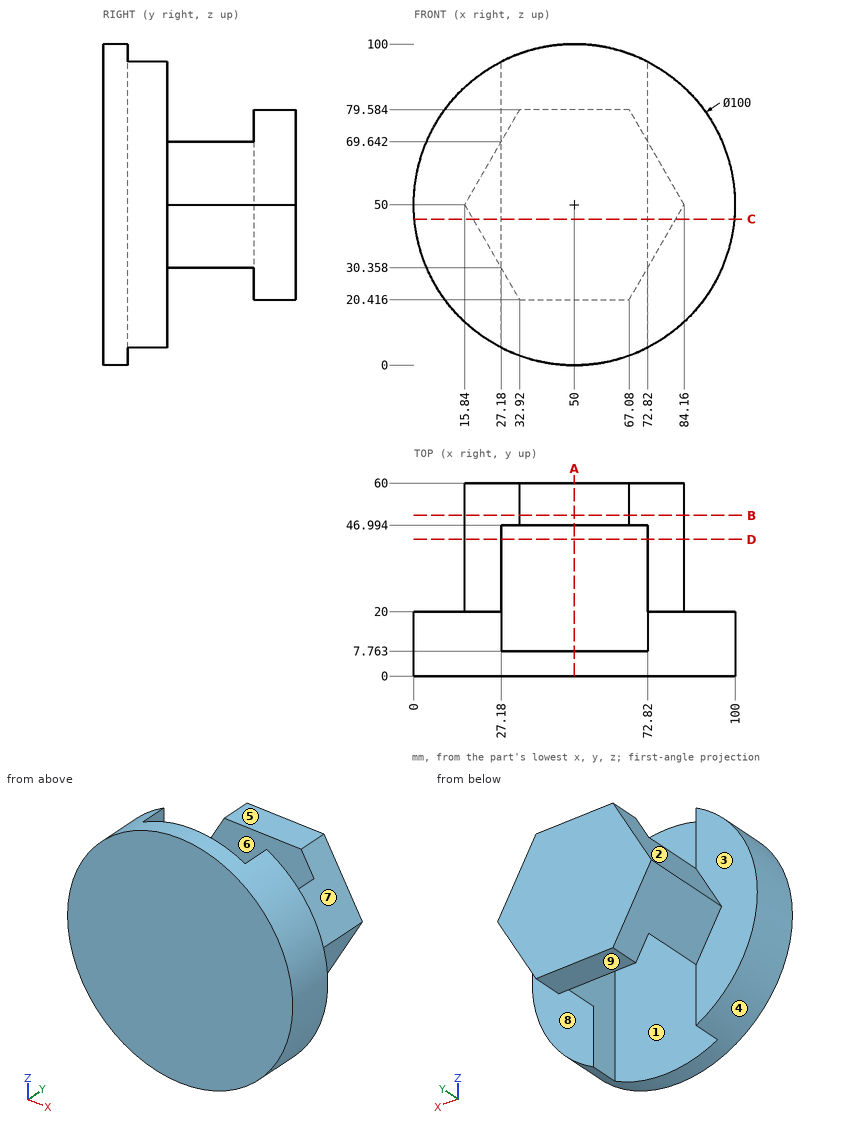
Job drawing, mm, ordinate dimensions from the low corner. One solid piece. A direction names the side the tool comes from. Give positions to 0.01 mm unless a question says otherwise; leave off trailing zeros. Loops run counter-clockwise (first coordinate to the right, second up) from the corner with the lowest first, then second, coordinate; pieces in that order, holes last. Notation, with made-up numbers: (12.25, 36.5) -> (44.25, 36.5) arc R20 ccw to (44.25, 69.5) -> close; hole circle Ø8 at (36, -29.75). An arc over 180 degrees is marked (long way). Write each question's results on one line, items separated by ' | '. Start each with the question number.
Q1. Band-saw the part on C-C on z = 45.5. List the corners of the cut face in (x, y), plus the area to 3 significant figures.
Q2. Band-saw the part on A-A on x = 50. List the corners of the cut face in (y, z), plus the area to 3 significant figures.
Q3. Pull direction X, two halves, no side cores. Call the marked faces 1, 2, 3 and 4: +X half, -X half, draft (parallel to the pull), parting line (faces both ways), or undercut.
Q4. Band-saw the part on D-D on y = 42.5. List the corners of the cut face in (x, z).
Q5. Wall check: L1, parallel to Y at x = 43, z = 62.5; L2, parallel to X at y = 16, z = 50; L3, parallel to Y at x = 46.5, z = 92. Give the ranges that are in metal, low to high.
Q6. Band-saw the part on B-B on y = 50. List the corners of the cut face in (x, z), plus the area to 3 significant figures.
Q7. Which spindle directions (+Z, -Z, +X, -X, +Y, -Y) get a long thin tool onto all of the face, cutting with end or side? Do the marked faces 5, 6, 7, 8 and 9. Say none if no direction does.
Q8. Pin check, flat tips, straight feed: P1, Ø1.5, axis at x = 73, z = 16, coming from the +Y side; P2, Ø12, axis at x = 17.5, y = 30.5, coming from the +Z side (1 decimal); P3, Ø4, axis at x = 50.5, y = 55, coming from the -Z side. Stop position of each tip, or through.
Results are:
1) outline: (0.2, 0) -> (99.8, 0) -> (99.8, 20) -> (81.56, 20) -> (81.56, 60) -> (18.44, 60) -> (18.44, 20) -> (0.2, 20) -> close; hole (27.18, 7.76) -> (72.82, 7.76) -> (72.82, 46.99) -> (27.18, 46.99) -> close | area: 2,730 mm²
2) outline: (0, 0) -> (7.76, 0) -> (7.76, 100) -> (0, 100) -> close; (46.99, 20.42) -> (60, 20.42) -> (60, 79.58) -> (46.99, 79.58) -> close | area: 1,550 mm²
3) face 1: undercut | face 2: -X half | face 3: draft | face 4: parting line
4) outline: (15.84, 50) -> (27.18, 30.36) -> (27.18, 69.64) -> close; (72.82, 30.36) -> (84.16, 50) -> (72.82, 69.64) -> close
5) L1: y = 0 to 7.76, 46.99 to 60 | L2: x = 0 to 27.18, 72.82 to 100 | L3: y = 0 to 7.76
6) outline: (15.84, 50) -> (32.92, 20.42) -> (67.08, 20.42) -> (84.16, 50) -> (67.08, 79.58) -> (32.92, 79.58) -> close | area: 3,030 mm²
7) face 5: +Z, +X, -X, +Y | face 6: +Z, -Z | face 7: +Z, +X, +Y | face 8: +X, +Y | face 9: -Z, +X, -X, +Y
8) P1: stops at y = 20 | P2: stops at z = 63.3 | P3: stops at z = 20.42
